Autodesk Inventor part; units mm, degrees
ref_plane "YZ Plane" through (0, 0, 0) normal (1, 0, 0) x (0, 1, 0)
ref_plane "XZ Plane" through (0, 0, 0) normal (0, 1, 0) x (-1, 0, 0)
ref_plane "XY Plane" through (0, 0, 0) normal (0, 0, 1) x (1, 0, 0)
sketch "Sketch1" plane through (0, 0, 0) normal (0, 0, 1) x (1, 0, 0)
  circle A0 centre (0, 0) radius 61
  arc A1 (7.0788, 15.7662) -> (7.8803, 16.1398) centre (0, 32) ccw
  circle A2 centre (0, 0) radius 61
  circle A3 centre (0, 32) radius 2.5
  circle A4 centre (0, 0) radius 50
  circle A5 centre (0, 0) radius 57.5 construction
  circle A6 centre (0, 0) radius 57 construction
  circle A7 centre (0, 0) radius 7.5 construction
  circle A8 centre (0, 32) radius 23 construction
  circle A9 centre (0, 0) radius 45 construction
  circle A10 centre (0, 32) radius 27.5 construction
  line L0 (-5.8547, -4.6875) -> (-21.4672, 14.8125) construction
  line L1 (5.8547, -4.6875) -> (21.4672, 14.8125) construction
  line L2 (0, 0) -> (0, 32) construction
  line L3 (7.5, 44.3706) -> (7.5, -44.3706) construction
  line L4 (-7.5, 44.3706) -> (-7.5, -44.3706) construction
  circle A11 centre (0, 0) radius 2.5
  line L5 (0, 0) -> (0, -15) construction
  circle A12 centre (0, -15) radius 2.5
  line L6 (-2.5, 0) -> (-2.5, -15)
  line L7 (2.5, -15) -> (2.5, 0)
  circle A13 centre (0, -7.5) radius 10 construction
  line L8 (-10, -7.5) -> (-10, 60.1747)
  line L9 (10, -7.5) -> (10, 60.1747)
  line L10 (-10, -7.5) -> (-10, -60.1747)
  line L11 (10, -7.5) -> (10, -60.1747)
  circle A14 centre (0, 0) radius 4
  circle A15 centre (0, -6.5) radius 2.5
  line L12 (0, -15) -> (0, -25)
  circle A16 centre (0, -25) radius 2.5
  point P0 (35.0374, 41.2549)
  point P1 (15.3046, 2.7982)
  point P2 (-19.4282, 41.2549)
  point P3 (0.3046, 2.7982)
  point P4 (25.4129, 52.2276)
  point P5 (-9.8037, 52.2276)
  point P6 (-10, 48.9898)
  point P7 (-10, -48.9898)
  point P8 (10, 48.9898)
  point P9 (10, -48.9898)
  point P10 (-2.5, -6.5)
  point P11 (2.5, -6.5)
  point P12 (-2.5, -3.1225)
  point P13 (2.5, -3.1225)
  dimension "d0" = 5
  dimension "d1" = 100
  dimension "d2" = 115
  dimension "d3" = 15
  dimension "d4" = 46
  dimension "d5" = 90
  dimension "d6" = 55
  dimension "d7" = 32
  dimension "d8" = 5
  dimension "d9" = 15
  dimension "d10" = 5
  dimension "d23" = 122
  dimension "d26" = 8
  dimension "d28" = 10
  dimension "d29" = 5
extrude "Extrusion1" add sketch "Sketch1" along normal blind 4 contours A0 L11 A4 L9 | L9 A4 L8 A0 | A0 L10 A4 L11 | L8 A4 L10 A0 | L9 L11 A4 L10 L8 | A16 | L7 A15 A14 | A14 A15 L6 | A15 | L7 A12 L6 A15 | A12
extrude "Extrusion2" add sketch "Sketch1" along normal blind 14 contours A16 | A15 | L7 A12 L6 A15 | A12
ref_plane "Work Plane1" through (0, -48.9898, 0) normal (1, 0, 0) x (0, 0, -1)
sketch "Sketch2" plane through (0, -48.9898, 0) normal (1, 0, 0) x (0, 0, -1)
  line L0 (-4, 109.9898) -> (-4, -12.0102)
  line L1 (0, 109.9898) -> (0, -12.0102)
  line L2 (0, 109.9898) -> (0, -12.0102)
  line L3 (0, -12.0102) -> (-10.3897, -12.0102)
  line L4 (-14, 33.9898) -> (-14, 31.4898)
  line L5 (0, -12.0102) -> (-4, -12.0102)
  line L6 (-4, -12.0102) -> (-4, -18.0102)
  line L7 (-2.6151, -18.0102) -> (0, -18.0102)
  line L8 (0, -18.0102) -> (0, -12.0102)
  line L9 (-5.1876, -17.2977) -> (-10.9042, -13.8677)
  arc A0 (-10.3897, -12.0102) -> (-10.9042, -13.8677) centre (-10.3897, -13.0102) ccw
  arc A1 (-5.1876, -17.2977) -> (-2.6151, -18.0102) centre (-2.6151, -13.0102) ccw
  line L10 (-0.0174, 48.9898) -> (-14.0174, 48.9898) construction
  line L11 (-0.0174, 48.9898) -> (13.9826, 48.9898) construction
  point P0 (0, 48.9898)
  point P1 (-14, -12.0102)
  dimension "d15" = 14
  dimension "d16" = 4
  dimension "d17" = 6
  dimension "d18" = 1
  dimension "d19" = 5
  dimension "d20" = 14
  dimension "d21" = 180
revolve "Revolution1" add sketch "Sketch2" angle 360 about axis through (0, 0, 0.0174) along (0, 0, 1)
properties part number "Gear Holder 2"
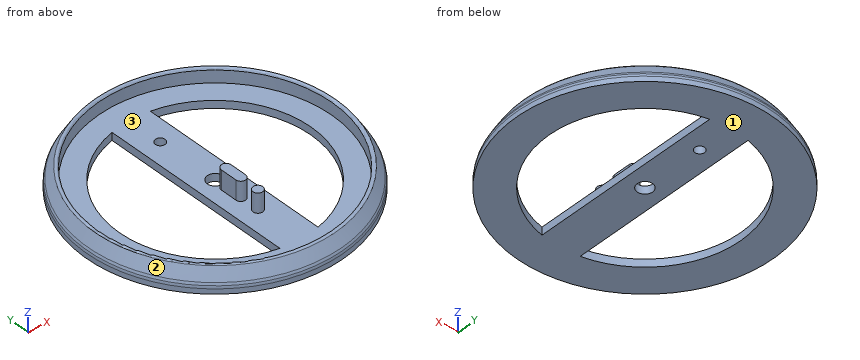
Could you check a few things on this model? Use its own coordinates, in mm. Face numbers are marked on the shaded views. Round coordinates to 2 decimals unless told otherwise and drop trailing zeros. Loops run counter-clockwise (first coordinate to the right, second up) from the corner with the lowest first, then second, coordinate; pieces in that order, holes last. Notation, with made-up numbers: (72.5, 51.25) - (89.5, 51.25) arc R16 cw to (89.5, 65.25) - close; hole circle Ø7 at (38.5, 37.5). An arc over 180 degrees is marked (long way). Write item = value, one per line.
1) I need wall thicknesses on line 1 along X through (y, z) = (24.5, 2.75); line 2 along X through (y, z) = (-39, 1.5); line 3 along Z through (x, y) = (51.5, -36). Which ranges of each line are inside material? Lowest first, please. Write a range as from..to.
Computed:
line_1 = -62.36..-43.59, -10..10, 43.59..62.36
line_2 = -54.48..-31.29, -10..10, 31.29..54.48
line_3 = 0..10.94
2) I'm going to push flat-ended pins straight in: P1, Ø4, axis at y = -10.5, z = 9.5, coming from the +X side; P2, Ø12, axis at x = -11, y = -31.5, coming from the +Z side; P3, Ø2, axis at x = -33.5, z = 8, coming from the -Y side. Where does each tip first touch, or does it pass through?
Computed:
P1 = 64.09
P2 = 4
P3 = -56.15
3) If we mould it in two halves opening along Y, with no side actions, what happens to the marked faces 1, 2 and 3? For each: pulls with the +Y half, pulls with the -Y half, needs draft (parallel to the pull), parting line crosses it, or undercut.
Computed:
face_1 = needs draft
face_2 = parting line crosses it
face_3 = undercut
4) Imagine slicing it at C-C (y = -25). Give the number of separate pieces and of enclosed holes in the cut face, and give its area (3 significant figures).
Computed:
separate_pieces = 3
enclosed_holes = 0
area = 341 mm2
5) Imagine slicing it at B-B (y = 0). Please give me the cut outline in (x, z), and give its area (3 significant figures).
Computed:
outline = (-67, 0) - (-50, 0) - (-50, 4) - (-61, 4) - (-61, 10.39) arc R1 ccw to (-62.86, 10.9) - (-66.29, 5.19) arc R5 ccw to (-67, 2.62) - close; (-10, 0) - (-4, 0) - (-4, 4) - (-10, 4) - close; (4, 0) - (10, 0) - (10, 4) - (4, 4) - close; (50, 0) - (67, 0) - (67, 2.62) arc R5 ccw to (66.29, 5.19) - (62.86, 10.9) arc R1 ccw to (61, 10.39) - (61, 4) - (50, 4) - close
area = 239 mm2
6) Imagine slicing it at A-A (z = 7.25). Please give me the cut outline in (x, y), and give its area (3 significant figures).
Computed:
outline = circle Ø130.1 at (0, 0); circle Ø5 at (0, -25); (-2.5, -15) arc R2.5 ccw to (2.5, -15) - (2.5, -6.5) arc R2.5 ccw to (-2.5, -6.5) - close; hole circle Ø122 at (0, 0)
area = 1,690 mm2
